Autodesk Fusion 360 part; units mm, degrees
sketch "Sketch1" plane through (0, 0, 0) normal (0, 0, 1) x (1, 0, 0)
  line L0 (-50, -50) -> (50, -50)
  line L1 (50, -50) -> (50, 50)
  line L2 (50, 50) -> (-50, 50)
  line L3 (-50, 50) -> (-50, -50)
  dimension "d1" = 100
  dimension "d2" = 100
  dimension "d3" = 50
  dimension "d4" = 50
extrude "Extrude1" add sketch "Sketch1" along normal blind 50
sketch "Sketch2" plane through (0, -50, 0) normal (0, -1, 0) x (1, 0, 0)
  line L0 (-50, 0) -> (50, 0)
  line L1 (50, 0) -> (50, 50)
  line L2 (50, 50) -> (-50, 50)
  line L3 (-50, 50) -> (-50, 0)
  line L4 (-46, 46) -> (46, 46)
  line L5 (46, 46) -> (46, 4)
  line L6 (46, 4) -> (-46, 4)
  line L7 (-46, 4) -> (-46, 46)
  dimension "d7" = 92
  dimension "d8" = 46
  dimension "d10" = 4
  dimension "d58" = 4
extrude "Extrude2" cut sketch "Sketch2" against normal blind 92 contours L4 L5 L6 L7
sketch "Sketch4" plane through (0, 0, 50) normal (0, 0, 1) x (-1, 0, 0)
  line L0 (50, -50) -> (50, 50)
  line L1 (50, 50) -> (-50, 50)
  line L2 (-50, 50) -> (-50, -50)
  line L3 (-50, -50) -> (50, -50)
  circle A0 centre (0, 0) radius 6
  dimension "d23" = 12
hole "Hole1" at (0, 0, 50) direction (0, 0, -1) diameter 20 depth 4 tip angle 118
fillet "Fillet2" radius 3.5 3 edges at (0, 42, 4) (-46, -4, 4) (46, -4, 4)
fillet "Fillet4" radius 2 3 edges at (-46, -4, 46) (0, 42, 46) (46, -4, 46)
sketch "Sketch10" plane through (0, 0, 0) normal (0, 0, -1) x (1, 0, 0)
  line L0 (-50, 50) -> (-50, -50)
  line L1 (-50, -50) -> (50, -50)
  line L2 (50, -50) -> (50, 50)
  line L3 (50, 50) -> (-50, 50)
  line L4 (-17.5, 17.5) -> (17.5, 17.5)
  line L5 (17.5, 17.5) -> (17.5, -17.5)
  line L6 (17.5, -17.5) -> (-17.5, -17.5)
  line L7 (-17.5, -17.5) -> (-17.5, 17.5)
  dimension "d105" = 35
  dimension "d106" = 35
  dimension "d107" = 17.5
  dimension "d108" = 17.5
extrude "Extrude8" add sketch "Sketch10" along normal blind 9 draft 32 contours L4 L5 L6 L7
sketch "Sketch12" plane through (0, 0, -9) normal (0, 0, -1) x (1, 0, 0)
  line L0 (-23.1238, 23.1238) -> (-23.1238, -23.1238)
  line L1 (-23.1238, -23.1238) -> (23.1238, -23.1238)
  line L2 (23.1238, -23.1238) -> (23.1238, 23.1238)
  line L3 (23.1238, 23.1238) -> (-23.1238, 23.1238)
  line L4 (-21.75, 21.75) -> (21.75, 21.75)
  line L5 (21.75, 21.75) -> (21.75, -21.75)
  line L6 (21.75, -21.75) -> (-21.75, -21.75)
  line L7 (-21.75, -21.75) -> (-21.75, 21.75)
  dimension "d111" = 43.5
  dimension "d112" = 43.5
  dimension "d113" = 21.75
  dimension "d114" = 21.75
extrude "Extrude9" cut sketch "Sketch12" against normal blind 9
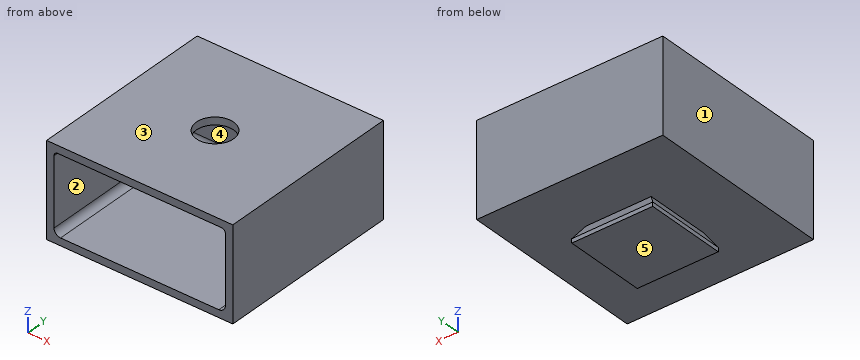
Could you check a few things on this model? Use its own coordinates, in mm. Face numbers are marked on the shaded views. A direction names the side the tool comes from. Coordinates: 2 decimals unless noted, no trailing zeros. Order: outer loops, then holes, each group sorted by start corner. A loop starts at its lowest first (then second) coordinate and runs counter-clockwise, first axis right, second up. Notation, with made-up numbers: M 32.5,3 L 79.5,3 A14 ccw 79.5,17 Z; hole C 58,-25 d2. An arc over 180 degrees is marked long. Use a Markdown table: item, result. Add a question column.
Q1. If I drill on L1, parallel to X at y = -26.5, z = 24; L2, parallel to Y at x = 0, z = 46.85, over which ranges is the centre line in solid material (lowest first)?
Q2. I want a section at B-B on z = 28.5. List the corners of the cut face in (x, y) for me, then the cut area to 3 significant figures.
Q3. I want a section at D-D on y = 0. List the corners of the cut face in (x, z) for me, then the cut area to 3 significant figures.
Q4. I want a section at C-C on y = -25.5. List the corners of the cut face in (x, z) for me, then the cut area to 3 significant figures.
Q5. We'd pull the mould along Z, two halves only. Please class the marked faces 1, 2 and 3: pulls with the +Z half, pulls with the -Z half, needs draft (parallel to the pull), parting line crosses it, or undercut.
Q6. I want a section at A-A on x = 0. List the corners of the cut face in (y, z) for me.
Q7. Which directions (+Z, -Z, +X, -X, +Y, -Y) give clear straight access to the entire face, cutting with the end or side of a thin tool? Please do the marked faces 4 and 5.
Q8. I'm going to push flat-ended pins straight in: pin 1 (6 mm diameter, centred on x = -4.5, z = 21, fed in from -Y); pin 2 (0.7 mm diameter, centred on y = 8, z = -8, fed in from -X); pin 3 (2.5 mm diameter, centred on x = 2, z = -8, fed in from -Y); pin 4 (4 mm diameter, centred on x = 7.5, z = -1, fed in from -Y). Where does each tip first touch, or does it pass through?
Checked values:
| question | item | result |
|---|---|---|
| 1 | L1 | -50 to -46, 46 to 50 |
| 1 | L2 | -50 to -10, 10 to 50 |
| 2 | outline | M -50,-50 L -46,-50 L -46,42 L 46,42 L 46,-50 L 50,-50 L 50,50 L -50,50 Z |
| 2 | area | 1,540 mm² |
| 3 | outline | M -50,0 L -17.5,0 L -21.75,-6.8 L -21.75,-9 L 21.75,-9 L 21.75,-6.8 L 17.5,0 L 50,0 L 50,50 L 10,50 L 10,46 L 44,46 A2 cw 46,44 L 46,7.5 A3.5 cw 42.5,4 L -42.5,4 A3.5 cw -46,7.5 L -46,44 A2 cw -44,46 L -10,46 L -10,50 L -50,50 Z |
| 3 | area | 1,430 mm² |
| 4 | outline | M -50,0 L 50,0 L 50,50 L -50,50 Z; hole M -46,7.5 A3.5 ccw -42.5,4 L 42.5,4 A3.5 ccw 46,7.5 L 46,44 A2 ccw 44,46 L -44,46 A2 ccw -46,44 Z |
| 4 | area | 1,140 mm² |
| 5 | face 1 | needs draft |
| 5 | face 2 | undercut |
| 5 | face 3 | pulls with the +Z half |
| 6 | outline | M -50,0 L -17.5,0 L -21.75,-6.8 L -21.75,-9 L 21.75,-9 L 21.75,-6.8 L 17.5,0 L 50,0 L 50,50 L 10,50 L 10,46 L 40,46 A2 cw 42,44 L 42,7.5 A3.5 cw 38.5,4 L -50,4 Z; M -50,46 L -10,46 L -10,50 L -50,50 Z |
| 7 | face 4 | -Y |
| 7 | face 5 | -Z, +X, -X, +Y, -Y |
| 8 | pin 1 | y = 42 |
| 8 | pin 2 | x = -21.75 |
| 8 | pin 3 | y = -21.75 |
| 8 | pin 4 | y = -50 |
